Build history of the part. All positions in model axes, mm. Face numbers are marked on the shaded views. A direction names the side the tool comes from. Coordinates: 2 decimals unless noted, no trailing zeros. Order: outer loops, then holes, each group sorted by start corner. A loop starts at its lowest first (then second) coordinate and runs counter-clockwise, first axis right, second up. Notation, with made-up numbers: (89.5, 86) - (134.5, 86) arc R21 ccw to (134.5, 95) - close; hole circle Ø3 at (14.25, -34). An arc over 180 degrees is marked (long way). One line per item, written item: value.
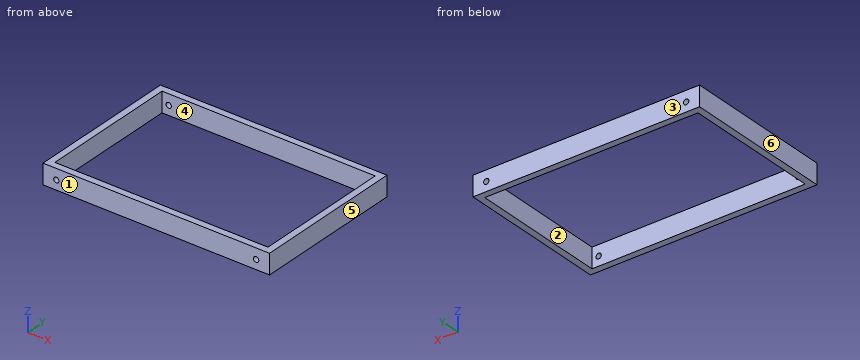
Autodesk Fusion 360 part; units mm, degrees
sketch "jig" plane through (0, 0, 0) normal (0, 0, 1) x (1, 0, 0)
  line L0 (-150, 0) -> (20, 0)
  line L1 (-150, 0) -> (-150, 116)
  line L2 (-150, 116) -> (20, 116)
  line L3 (20, 116) -> (20, 0)
  line L4 (-144.988, 5.0299) -> (15.012, 5.0299)
  line L5 (-144.988, 5.0299) -> (-144.988, 111.0299)
  line L6 (15.012, 5.0299) -> (15.012, 111.0299)
  line L7 (15.012, 111.0299) -> (-144.988, 111.0299)
  dimension "d1" = 170
  dimension "d2" = 116
  dimension "d3" = 170
  dimension "d4" = 160
  dimension "d5" = 106
  dimension "d6" = 106
extrude "Extrude1" add sketch "jig" along normal blind 10
extrude "Extrude2" add 1 faces at (-91.6627, 1.6766, 10) along direction (0, 0, 1) blind 5
sketch "bolt holes" plane through (0, 0, 0) normal (0, 1, 0) x (1, 0, 0)
  circle A0 centre (10, -7) radius 2
  circle A1 centre (-140, -7) radius 2
  dimension "d11" = 4
  dimension "d12" = 4
extrude "Extrude3" cut sketch "bolt holes" along normal blind 130 contours A1
extrude "Extrude4" cut sketch "bolt holes" along normal blind 140 contours A0
extrude "Extrude5" add 1 faces at (-40.4634, 111.0299, 12.8047) along direction (0, -1, 0) blind 3
extrude "Extrude6" cut 1 faces at (-147.3309, 116, 7.3899) along direction (0, -1, 0) blind 3
extrude "Extrude7" add 1 faces at (-147.3309, 113, 7.3899) along direction (0, 1, 0) blind 1
extrude "Extrude8" cut 1 faces at (-40.4634, 108.0299, 12.8047) along direction (0, 1, 0) blind 1
1. 3-axis set-ups, long thin cutter, end or side, ignore diameter. For the marked faces 1 and 2: which of +Z, -Z, +X, -X, +Y, -Y reach the whole face in a straight line?
Values found:
face 1: +Z, -Z, +X, -X, -Y
face 2: +Z, -Z
2. Band-saw the part on D-D, the plane x = -64.5. Give the cut face in (y, z), and give its area (3 significant figures).
Values found:
outline: (0, 0) - (5.03, 0) - (5.03, 15) - (0, 15) - close; (109.03, 0) - (114, 0) - (114, 15) - (109.03, 15) - close
area: 150 mm2
3. Band-saw the part on B-B, the plane z = 13. Give the cut face in (x, y), and give its area (3 significant figures).
Values found:
outline: (-150, 0) - (20, 0) - (20, 114) - (-150, 114) - close; hole (-144.99, 5.03) - (15.01, 5.03) - (15.01, 109.03) - (-144.99, 109.03) - close
area: 2,740 mm2
4. Band-saw the part on A-A, the plane x = -140. Give the cut face in (y, z).
Values found:
outline: (0, 0) - (5.03, 0) - (5.03, 5) - (0, 5) - close; (0, 9) - (5.03, 9) - (5.03, 15) - (0, 15) - close; (109.03, 0) - (114, 0) - (114, 5) - (109.03, 5) - close; (109.03, 9) - (114, 9) - (114, 15) - (109.03, 15) - close
5. Band-saw the part on C-C, the plane y = 104. Give the cut face in (x, z).
Values found:
outline: (-150, 0) - (-144.99, 0) - (-144.99, 15) - (-150, 15) - close; (15.01, 0) - (20, 0) - (20, 15) - (15.01, 15) - close
6. Probe line 1 along X through (y, z) = (34.5, 3.75); line 2 along Z through (x, y) = (10, 1.1); line 3 along Y through (x, z) = (-66, 7.25). List the from-to ranges inside material, lowest first.
Values found:
line 1: x = -150 to -144.99, 15.01 to 20
line 2: z = 0 to 5, 9 to 15
line 3: y = 0 to 5.03, 109.03 to 114
7. Two-plate mould, pull along X, no slides. Class the marked faces 3, 4, 5 and 6: pulls with the +X half, pulls with the -X half, needs draft (parallel to the pull), parting line crosses it, or undercut.
Values found:
face 3: needs draft
face 4: undercut
face 5: pulls with the +X half
face 6: pulls with the -X half
